Read the model definition and answer for the solid it produces. Units are mm, in the model's axes. A direction names the side the tool comes from. Coordinates: 2 decimals unless noted, no trailing zeros. Write each loop counter-clockwise with the first axis right and the second up, starting at its lowest first coordinate (ties: lowest second). Pieces come first, ordered by that corner, then holes. Notation, with made-up numbers: M -5,-27.5 L 6,-27.5 A20 cw 6,-19.5 Z; hole C -34,-7 d2. An arc over 180 degrees is marked long. Write item = value, one per line.
from build123d import *

# Parameters (mm, degrees)
SKETCH1_W                                     = 38.1
SKETCH1_H                                     = 38.1
BOSS_EXTRUDE1_DEPTH                           = 9.525
SKETCH4_R                                     = 4.7625
CUT_EXTRUDE1_DEPTH                            = 44.649033494
MOTORHOLES_D                                  = 2.2606
CBORE_FOR_6_SOCKET_HEAD_CAP_SCREW1_AT_2_COUNT = 2
CBORE_FOR_6_SOCKET_HEAD_CAP_SCREW1_AT_2_PITCH = 25.4
CHAMFER1_SIZE                                 = 10.16


with BuildPart() as part:
    # Sketch1 → Boss-Extrude1 (new body)
    with BuildSketch(Plane(origin=(0, 0, 0), x_dir=(1, 0, 0), z_dir=(0, 1, 0))):
        Rectangle(SKETCH1_W, SKETCH1_H)
    extrude(amount=BOSS_EXTRUDE1_DEPTH)

    # Sketch4 → Cut-Extrude1 (cut, through all)
    with BuildSketch(Plane.XY.offset(19.05)):
        with Locations((0, 9.525)):
            Circle(SKETCH4_R)
    extrude(amount=-CUT_EXTRUDE1_DEPTH, mode=Mode.SUBTRACT)

    # MotorHoles (through all)
    with Locations(Plane(origin=(0, 0, 0), x_dir=(-1, 0, 0), z_dir=(0, -1, 0))):
        with Locations((-5.715, -15.875), (5.715, -15.875)):
            Hole(MOTORHOLES_D / 2)

    # Sketch5 → CBORE for #6 Socket Head Cap Screw1 (revolve, cut)
    with BuildSketch(Plane(origin=(12.7, 0, -9.525), x_dir=(0, 0, -1), z_dir=(1, 0, 0))):
        Polygon((0, 0), (0, 9.525), (1.8288, 9.525), (1.8288, 3.5052), (3.57251, 3.5052), (3.57251, 0.635), (4.20751, 0), align=None)
    cbore_for_6_socket_head_cap_screw1 = revolve(axis=Axis((12.7, -6.35, -9.525), (0, 1, 0)), mode=Mode.SUBTRACT)

    # CBORE for #6 Socket Head Cap Screw1 at 2: CBORE for #6 Socket Head Cap Screw1 ×2
    with Locations(*[(-i * CBORE_FOR_6_SOCKET_HEAD_CAP_SCREW1_AT_2_PITCH, 0, 0) for i in range(1, CBORE_FOR_6_SOCKET_HEAD_CAP_SCREW1_AT_2_COUNT)]):
        add(cbore_for_6_socket_head_cap_screw1, mode=Mode.SUBTRACT)

    # Chamfer1
    chamfer1_edges = [part.edges().sort_by_distance(p)[0] for p in [
        (19.05, 4.7625, 19.05),
        (-19.05, 4.7625, 19.05),
    ]]
    chamfer(chamfer1_edges, length=CHAMFER1_SIZE)


solid = part.part
Item 1: For a pull along Z with two mould halves and no side action, classify faces 3 (the face through (14.04, 4.7, 13.9)), 4 (the face through (-19.05, 5, -5)), 5 (the face through (14, 3.505, -8)) as released by +Z, released by -Z, zero draft, split by the parting line, or undercut.
Worked answers:
face_3 = released by +Z
face_4 = zero draft
face_5 = undercut
Item 2: Find section D-D (y = 4). Determine the outline of the cut face in (x, z) (3 decimals).
Worked answers:
outline = M -19.05,-19.05 L 19.05,-19.05 L 19.05,8.89 L 8.89,19.05 L -8.89,19.05 L -19.05,8.89 Z; hole C -12.7,-9.525 d3.658; hole C -5.715,15.875 d2.261; hole C 5.715,15.875 d2.261; hole C 12.7,-9.525 d3.658
Item 3: A flat-ended cylindrical pin translates along its axis: pin 1 (2 mm diameter, centred on x = 14, z = -9, fed in from -Y). Find the tip coordinate at first contact, or state that the pin passes through.
Worked answers:
pin_1 = 3.51
Item 4: Find section B-B (y = 7.25). Determine the outline of the cut face in (x, z) (3 decimals).
Worked answers:
outline = M -19.05,-19.05 L -4.184,-19.05 L -4.184,19.05 L -8.89,19.05 L -19.05,8.89 Z; M 4.184,-19.05 L 19.05,-19.05 L 19.05,8.89 L 8.89,19.05 L 4.184,19.05 Z; hole C -12.7,-9.525 d3.658; hole C -5.715,15.875 d2.261; hole C 5.715,15.875 d2.261; hole C 12.7,-9.525 d3.658
Item 5: Consider line 1 along X through (y, z) = (7.75, -10); line 2 along X through (y, z) = (0.5, 16); line 3 along Z through (x, y) = (-12.7, 5.25). Determine where each line is inside the solid, lowest interval first. Write a range as from..to.
Worked answers:
line_1 = -19.05..-14.47, -10.93..-4.42, 4.42..10.93, 14.47..19.05
line_2 = -11.94..-6.84, -4.59..4.59, 6.84..11.94
line_3 = -19.05..-11.35, -7.7..15.24
Item 6: Which of the six approach directions +Z, -Z, +X, -X, +Y, -Y give full straight-line access (tool end or side, diameter ignored) to faces 1 (the face through (12, 9.525, 0)), 2 (the face through (-11, 3.505, -8))?
Worked answers:
face_1 = +Z, -Z, +X, -X, +Y
face_2 = -Y
Item 7: Find section C-C (z = 11.5). Determine the outline of the cut face in (x, y) (1 decimal), and give its area (3 significant figures).
Worked answers:
outline = M -16.4,0 L 16.4,0 L 16.4,9.5 L 4.8,9.5 A4.8 cw -4.8,9.5 L -16.4,9.5 Z
area = 278 mm²
